Autodesk Inventor part; units mm, degrees
ref_plane "YZ Plane" through (0, 0, 0) normal (1, 0, 0) x (0, 1, 0)
ref_plane "XZ Plane" through (0, 0, 0) normal (0, 1, 0) x (-1, 0, 0)
ref_plane "XY Plane" through (0, 0, 0) normal (0, 0, 1) x (1, 0, 0)
sketch "草图2" plane through (0, 0, 0) normal (0, 0, 1) x (1, 0, 0)
  circle A0 centre (8, 60) radius 2.1
  circle A1 centre (20, 60) radius 2.1
  circle A2 centre (20, 75) radius 2.1
  circle A3 centre (20, 90) radius 1.75
  circle A4 centre (8, 90) radius 2.1
  line L0 (22, 54) -> (0, 54)
  arc A5 (22, 54) -> (25, 57) centre (22, 57) ccw
  line L1 (25, 93) -> (25, 57)
  line L2 (0, 96) -> (22, 96)
  arc A6 (25, 93) -> (22, 96) centre (22, 93) ccw
  line L3 (0, 96) -> (-6.5, 96)
  line L4 (-6.5, 96) -> (-6.5, 54)
  line L5 (-6.5, 54) -> (0, 54)
  line L6 (0, 54) -> (0, 96)
  circle A7 centre (20, 60) radius 2.1
  circle A8 centre (8, 60) radius 2.1
  circle A9 centre (20, 75) radius 2.1
  circle A10 centre (20, 90) radius 2.1
  circle A11 centre (8, 90) radius 2.1
  point P0 (0, 0)
  dimension "d0" = 6.5
  dimension "d11" = 4.2
  dimension "d12" = 4.2
  dimension "d13" = 4.2
  dimension "d14" = 4.2
  dimension "d15" = 4.2
extrude "拉伸1" add sketch "草图2" along normal blind 3 contours L0 L6 L2 A6 L1 A5 | L5 L4 L3 L6
sketch "草图3" plane through (0, 0, 3) normal (0, 0, 1) x (1, 0, 0)
  line L0 (-6.5, 54) -> (22, 54)
  line L1 (22, 96) -> (-6.5, 96)
  line L2 (-6.5, 54) -> (-2.5, 54)
  line L3 (-2.5, 54) -> (-2.5, 96)
  line L4 (-2.5, 96) -> (-6.5, 96)
  line L5 (-6.5, 96) -> (-6.5, 54)
  point P0 (0, 0)
  dimension "d3" = 4
extrude "拉伸2" add sketch "草图3" along normal blind 25
fillet "圆角1" radius 5 1 edges at (-2.5, 75, 3)
fillet "圆角2" radius 5 2 edges at (-6.5, 96, 14) (-6.5, 54, 14)
properties part number "拖带架"
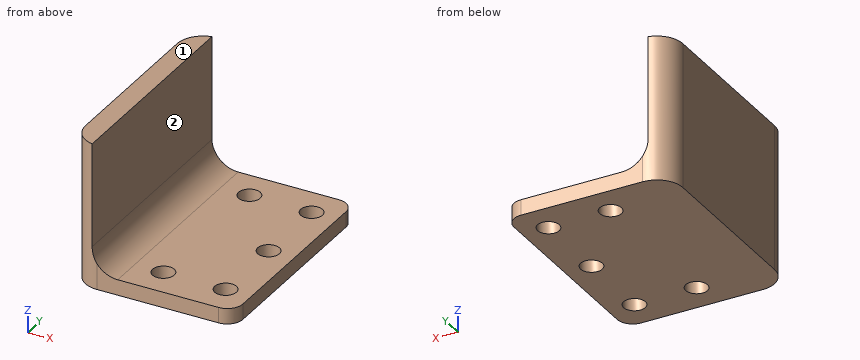
Design review of the part built by this model. Coordinates are the model's own, in mm. Face numbers are marked on the shaded views. A direction names the side the tool comes from. Give positions to 0.01 mm unless a question says otherwise; leave off trailing zeros. Order: outer loops, then holes, each group sorted by start corner. A loop starts at its lowest first (then second) coordinate and runs counter-clockwise, first axis right, second up. Notation, with made-up numbers: (30, -14.75) -> (52, -14.75) arc R25 cw to (52, 11.25) -> close; hole circle Ø6 at (-34.75, 41). An arc over 180 degrees is marked (long way). Write item = value, one per line. Start each with the question number.
(1) To check wall thickness, follow line 1 along Y through (x, z) = (20, 2); line 2 along Z through (x, y) = (8, 57); line 3 along X through (y, z) = (76.5, 26.75). State the ranges of each line that lie inside material, in increasing order.
(2) We need section B-B on y = 75. Write out the cut boundary in (x, z).
(3) We need section C-C on x = 20. Write out the cut boundary in (y, z), plus the area to 3 significant figures.
(4) For the marked faces 1 and 2, list the 3-axis set-ups (+Z, -Z, +X, -X, +Y, -Y) from which the entire face can be reached by the end or side of a thin tool; tool diameter is ignored.
(5) For pin 1 (10 mm diameter, centred on x = 4.5, y = 59.5, fed in from +Z); pin 2 (7 mm diameter, centred on x = 18, y = 83, fed in from +Z); pin 3 (3.5 mm diameter, centred on x = 8, y = 90, fed in from -Z); pin 4 (12 mm diameter, centred on x = 5, y = 89, fed in from +Z), all flat-tipped, find the tip position at first contact; note any pin that passes through.
(6) We need section D-D on y = 66. Write out the cut boundary in (x, z), plus the area to 3 significant figures.
(7) We need section A-A on x = 8. Write out the cut boundary in (y, z), plus the area to 3 significant figures.
Numbers:
q1.line_1 = 54 to 57.9, 62.1 to 72.9, 77.1 to 87.9, 92.1 to 96
q1.line_2 = 0 to 3
q1.line_3 = -6.5 to -2.5
q2.outline = (-6.5, 0) -> (17.9, 0) -> (17.9, 3) -> (2.5, 3) arc R5 cw to (-2.5, 8) -> (-2.5, 28) -> (-6.5, 28) -> close; (22.1, 0) -> (25, 0) -> (25, 3) -> (22.1, 3) -> close
q3.outline = (54, 0) -> (57.9, 0) -> (57.9, 3) -> (54, 3) -> close; (62.1, 0) -> (72.9, 0) -> (72.9, 3) -> (62.1, 3) -> close; (77.1, 0) -> (87.9, 0) -> (87.9, 3) -> (77.1, 3) -> close; (92.1, 0) -> (96, 0) -> (96, 3) -> (92.1, 3) -> close
q3.area = 88.2 mm^2
q4.face_1 = +Z, +X, -X, +Y, -Y
q4.face_2 = +Z, +X, +Y, -Y
q5.pin_1 = 4
q5.pin_2 = 3
q5.pin_3 = through
q5.pin_4 = 4.43
q6.outline = (-6.5, 0) -> (25, 0) -> (25, 3) -> (2.5, 3) arc R5 cw to (-2.5, 8) -> (-2.5, 28) -> (-6.5, 28) -> close
q6.area = 200 mm^2
q7.outline = (54, 0) -> (57.9, 0) -> (57.9, 3) -> (54, 3) -> close; (62.1, 0) -> (87.9, 0) -> (87.9, 3) -> (62.1, 3) -> close; (92.1, 0) -> (96, 0) -> (96, 3) -> (92.1, 3) -> close
q7.area = 101 mm^2
